from build123d import *

# Parameters (mm, degrees)
F2_SIZE = 0.5
F4_R    = 1


# Not quite as in the source:
# - a fillet or chamfer that OpenCascade refuses, or shapes differently, is made with other operations: its cross-section is extruded or revolved along the edge and cut away or added


with BuildPart() as f1:
    # F0 (on Front) → F1 (revolve)
    with BuildSketch(Plane.XZ):
        Polygon((23.2, 30), (21.2, 30), (21.2, 10), (18.2991344482, 10), (18.2991344482, 0), (0, 0), (0, -2), (52.7682006359, -2), (52.7682006359, 0), (26.7173200846, 0), align=None)
    revolve(axis=Axis((0, 0, 5.5142873898), (0, 0, -1)))

    # F2
    f2_edges = [f1.edges().sort_by_distance(p)[0] for p in [
        (-52.768201, 0, -2),
    ]]
    chamfer(f2_edges, length=F2_SIZE)

    # F3: fillet of radius 5 on 2 edges, made by hand

    # F3_s1 → F3_t2 (revolve)
    with BuildSketch(Plane.XZ):
        with BuildLine():
            ThreePointArc((31.1653481678, 0), (27.8420335373, 1.2642832191), (26.1993632745, 4.4177680532))
            Line((26.1993632745, 4.4177680532), (26.1000435766, 4.4061234142))
            Line((26.1000435766, 4.4061234142), (26.6283595229, -0.1))
            Line((26.6283595229, -0.1), (31.1653481678, -0.1))
            Line((31.1653481678, -0.1), (31.1653481678, 0))
        make_face()
    revolve(axis=Axis((0, 0, 0), (0, 0, -1)))

    # F3_s3 → F3_t4 (revolve, cut)
    with BuildSketch(Plane.XZ):
        with BuildLine():
            ThreePointArc((52.7682006359, -1.5), (51.1339780947, -0.3902277714), (49.1974864216, 0))
            Line((49.1974864216, 0), (49.1974864216, 0.1))
            Line((49.1974864216, 0.1), (52.7682006359, 0.1))
            Line((52.7682006359, 0.1), (52.8682006359, 0))
            ThreePointArc((52.8682006359, 0), (52.8682006359, -0.75), (52.8396149202, -1.43))
            Line((52.8396149202, -1.43), (52.7682006359, -1.5))
        make_face()
    revolve(axis=Axis((0, 0, 0), (0, 0, -1)), mode=Mode.SUBTRACT)

    # F4
    f4_edges = [f1.edges().sort_by_distance(p)[0] for p in [
        (-23.2, 0, 30),
    ]]
    fillet(f4_edges, radius=F4_R)


solid = f1.part
Source: CAD feature listing. Evaluate the final solid. Frame: model axes, mm. A direction names the side the tool comes from. Coordinates: 2 decimals unless noted, no trailing zeros. Loops run counter-clockwise (first coordinate to the right, second up) from the corner with the lowest first, then second, coordinate; pieces in that order, holes last. Notation, with made-up numbers: (67, 20) - (76, 20) arc R14 ccw to (76, 43) - close; hole circle Ø1 at (-4.75, 65). An arc over 180 degrees is marked (long way). Return JSON: item names as keys, results as strings.
Q1. Section C-C, the plane z = 17. Return loops of the section in (x, y), plus the area to 3 significant figures.
Results:
{"outline": "circle Ø49.45 at (0, 0); hole circle Ø42.4 at (0, 0)", "area": "508 mm2"}
Q2. Mould query, pull axis Y, two halves, no side actions, for faces 1 (the cylindrical face through (17.454, -5.497, 4.93)), 2 (the cylindrical face through (19.583, 8.12, 19.86)), 3 (the flat face through (-1, 32, 0)), 4 (the conical face through (-19.371, 14.853, 19.684)). Classes: released by +Y, released by -Y, zero draft, split by the parting line, or undercut.
Results:
{"face 1": "undercut", "face 2": "undercut", "face 3": "zero draft", "face 4": "split by the parting line"}
Q3. Contact query for flat-ended pins moving along their axis: P1, Ø8, axis at x = 13.5, z = 24, coming from the +Y side; P2, Ø6, axis at x = 25, z = 19.5, coming from the -Y side; P3, Ø8, axis at x = 0.5, z = 2, coming from the -Y side; P4, Ø8, axis at x = 29.5, z = 26, coming from the +Y side. Output: stop coordinate, or through.
Results:
{"P1": "y = 22.01", "P2": "y = -10.68", "P3": "y = -52.77", "P4": "through"}
Q4. Section A-A, the plane y = 0. Return loops of the section in (x, z).
Results:
{"outline": "(-52.77, -1.5) - (-52.27, -2) - (52.27, -2) - (52.77, -1.5) arc R5 ccw to (49.2, 0) - (31.17, 0) arc R5 cw to (26.2, 4.42) - (23.3, 29.12) arc R1 ccw to (22.31, 30) - (21.2, 30) - (21.2, 10) - (18.3, 10) - (18.3, 0) - (-18.3, 0) - (-18.3, 10) - (-21.2, 10) - (-21.2, 30) - (-22.31, 30) arc R1 ccw to (-23.3, 29.12) - (-26.2, 4.42) arc R5 cw to (-31.17, 0) - (-49.2, 0) arc R5 ccw to start"}
Q5. Material intervals for line 1 along X through (y, z) = (0, 3); line 2 along Y through (x, z) = (0, 2.75); line 3 along X through (y, z) = (12, 14), sorted ascending.
Results:
{"line 1": "-26.58 to -18.3, 18.3 to 26.58", "line 2": "-26.7 to -18.3, 18.3 to 26.7", "line 3": "-22.02 to -17.48, 17.48 to 22.02"}
Q6. Access query for faces 5 (the flat face through (20, 8, 30)), 6 (the flat face through (-17.4, 6.2, 10)). Directions: +Z, -Z, +X, -X, +Y, -Y. A direction counts if a zero-diameter tool reaches every point of the face in a straight line with its end or side. Return the directions, or none.
Results:
{"face 5": "+Z, +X, -X, +Y, -Y", "face 6": "+Z"}
Q7. Section D-D, the plane z = 23. Return loops of the section in (x, y), plus the area to 3 significant figures.
Results:
{"outline": "circle Ø48.04 at (0, 0); hole circle Ø42.4 at (0, 0)", "area": "401 mm2"}
